from build123d import *

# Parameters (mm, degrees)
SKETCH_1_R      = 6.5
EXTRUDE_2_DEPTH = 3
SKETCH_3_R      = 5.5
EXTRUDE_3_DEPTH = 5
FILLET_1_R      = 1
SKETCH_4_W      = 0.326388432
SKETCH_4_H      = 3.66280352
EXTRUDE_4_DEPTH = 1


with BuildPart() as part:
    # 草图1 → 凸台-拉伸2 (new body)
    with BuildSketch(Plane(origin=(0, 0, 0), x_dir=(1, 0, 0), z_dir=(0, 1, 0))):
        Circle(SKETCH_1_R)
    extrude(amount=EXTRUDE_2_DEPTH)

    # 草图3 → 凸台-拉伸3 (add)
    with BuildSketch(Plane(origin=(0, 3, 0), x_dir=(1, 0, 0), z_dir=(0, 1, 0))):
        Circle(SKETCH_3_R)
    extrude(amount=EXTRUDE_3_DEPTH)

    # 圆角1
    fillet_1_edges = [part.edges().sort_by_distance(p)[0] for p in [
        (-5.5, 8, 0),
    ]]
    fillet(fillet_1_edges, radius=FILLET_1_R)

    # 草图4 → 凸台-拉伸4 (add)
    with BuildSketch(Plane(origin=(0, 8, 0), x_dir=(1, 0, 0), z_dir=(0, 1, 0))):
        with BuildLine():
            Line((-2.843597496, 0), (-2.339117099, 0))
            ThreePointArc((-2.339117099, 0), (0, -2.339117099), (2.339117099, 0))
            Line((2.339117099, 0), (2.843597496, 0))
            ThreePointArc((2.843597496, 0), (0, -2.843597496), (-2.843597496, 0))
        make_face()
        with Locations((0, 0.924767225)):
            Rectangle(SKETCH_4_W, SKETCH_4_H)
    extrude(amount=EXTRUDE_4_DEPTH)


solid = part.part
Check sheet for the modelled part. Datum: model origin and axes. Units: mm. A direction names the side the tool comes from. Round coordinates to 2 decimals unless told otherwise and drop trailing zeros. Write each loop counter-clockwise with the first axis right and the second up, starting at its lowest first coordinate (ties: lowest second). Pieces come first, ordered by that corner, then holes. Notation, with made-up numbers: (55.5, 78) - (113.5, 78) arc R24 ccw to (113.5, 115) - close; hole circle Ø9 at (32.25, 81.5). An arc over 180 degrees is marked (long way). Return JSON: item names as keys, results as strings.
Q1. Scan lines: L1, parallel to Y at x = 2.5, z = -5.5; L2, parallel to Y at x = 1.25, z = 3.25; L3, parallel to X at y = 2, z = 2.25. Record each from-to range of solid material in increasing order. Write a range as from..to.
Returned:
{"L1": "y = 0..3", "L2": "y = 0..8", "L3": "x = -6.1..6.1"}
Q2. Cross-section at B-B (y = 2). Record the boundary of the cut face in (x, z).
Returned:
{"outline": "circle Ø13 at (0, 0)"}
Q3. Draft check along X on faces 4 (the cylindrical face through (0.063, 8.493, 2.843)), 5 (the flat face through (1, 8, 0)), 6 (the cylindrical face through (-0.05, 8.49, 2.34)), 7 (the flat face through (-5, 3, -3)). Enter one of: released by +X, released by -X, zero draft, split by the parting line, or undercut.
Returned:
{"face 4": "split by the parting line", "face 5": "undercut", "face 6": "undercut", "face 7": "zero draft"}
Q4. Cross-section at A-A (y = 5). Record the boundary of the cut face in (x, z).
Returned:
{"outline": "circle Ø11 at (0, 0)"}
Q5. Access from +Z, -Z, +X, -X, +Y, -Y to the whole of each face (thin tool, end or side, straight path). Record for faces 1 (the flat face through (0.163, 8.5, -0.9)), 2 (the cylindrical face through (-5.158, 1.479, 3.955)), 3 (the cylindrical face through (-1.19, 4.97, 5.37)).
Returned:
{"face 1": "-Z, +Y", "face 2": "+Y, -Y", "face 3": "+Y"}
Q6. Depth check by flat-ended pin: P1, Ø1, axis at x = 1.5, y = 2, coming from the -Z side; P2, Ø4, axis at x = -4.5, y = 4.5, coming from the +Z side. Enter the tip coordinate at first touch or a pass-through.
Returned:
{"P1": "stops at z = -6.42", "P2": "stops at z = 5.67"}
